```python
from build123d import *

# Parameters (mm, degrees)
SKETCH1_W           = 10
SKETCH1_H           = 10
BOSS_EXTRUDE1_DEPTH = 50
BOSS_EXTRUDE2_START = -45
SKETCH2_R           = 20
BOSS_EXTRUDE2_DEPTH = 2.5
FILLET2_R           = 2
FILLET3_R           = 5
FILLET4_R           = 5


with BuildPart() as part:
    # Sketch1 → Boss-Extrude1 (new, symmetric)
    with BuildSketch(Plane(origin=(0, 0, 0), x_dir=(1, 0, 0), z_dir=(0, 1, 0))):
        Rectangle(SKETCH1_W, SKETCH1_H)
    extrude(amount=BOSS_EXTRUDE1_DEPTH, both=True)

    # Sketch2 → Boss-Extrude2 (add, symmetric)
    with BuildSketch(Plane(origin=(0, 50, 0), x_dir=(1, 0, 0), z_dir=(0, 1, 0)).offset(BOSS_EXTRUDE2_START)):
        with Locations(Location((0, 0, 0), (0, 0, 270))):
            Circle(SKETCH2_R)
    extrude(amount=BOSS_EXTRUDE2_DEPTH, both=True)

    # Fillet2
    fillet2_edges = [part.edges().sort_by_distance(p)[0] for p in [
        (5, -23.75, 5),
        (-5, -23.75, 5),
        (-5, -23.75, -5),
        (5, -23.75, -5),
    ]]
    fillet(fillet2_edges, radius=FILLET2_R)

    # Fillet3
    fillet3_edges = [part.edges().sort_by_distance(p)[0] for p in [
        (-5, 28.75, -5),
        (-5, 28.75, 5),
        (5, 28.75, 5),
        (5, 28.75, -5),
    ]]
    fillet(fillet3_edges, radius=FILLET3_R - 0.0001)  # a hair under: the kernel refuses the full size

    # Fillet4
    fillet4_edges = [part.edges().sort_by_distance(p)[0] for p in [
        (3.535563195, 50, -3.535563195),
        (3.535563195, 50, 3.535563195),
        (-3.535563195, 50, 3.535563195),
        (-3.535563195, 50, -3.535563195),
    ]]
    fillet(fillet4_edges, radius=FILLET4_R - 0.0001)  # a hair under: the kernel refuses the full size


solid = part.part
```
Geometry: final body of the model. Coordinates: model frame, mm. A direction names the side the tool comes from. Round coordinates to 2 decimals unless told otherwise and drop trailing zeros. Write each loop counter-clockwise with the first axis right and the second up, starting at its lowest first coordinate (ties: lowest second). Pieces come first, ordered by that corner, then holes.
Item 1: Section query B-B (x = -16). Return loops of the section in (y, z), plus the area to 3 significant figures.
Item 2: Pin query (flat end, axial travel): P1, Ø1.8, axis at y = -31, z = 0.5, coming from the -X side; P2, Ø6.5, axis at x = -1, y = -13, coming from the -Z side; P3, Ø6.5, axis at y = -19, z = 1, coming from the +X side. Return the tip coordinate at first contact, or that it passes through.
Item 3: Material intervals for L1, parallel to X at y = -8.5, z = -1.5; L2, parallel to Y at x = 12, z = -9, sorted ascending.
Item 4: Set-up query: faces 1 (the face through (-4.43, -24.12, -4.4)), 2 (the face through (-4.43, -23.38, 4.4)), 3 (the face through (0, -23, -5)), 4 (the face through (-5, -23, 0)), 5 (the face through (-4, 26, -3)). Return all of +Z, -Z, +X, -X, +Y, -Y with unobstructed straight access to the full face (end or side cutting, diameter ignored); none if empty.
Item 5: Section query A-A (y = -39). Return loops of the section in (x, z).
Completed:
1. outline: (2.5, -12) - (7.5, -12) - (7.5, 12) - (2.5, 12) - close
1. area: 120 mm2
2. P1: stops at x = -5
2. P2: stops at z = -5
2. P3: stops at x = 5
3. L1: x = -5 to 5
3. L2: y = 2.5 to 7.5
4. face 1: -Z, -X, -Y
4. face 2: +Z, -X, -Y
4. face 3: -Z, +X, -X, -Y
4. face 4: +Z, -Z, -X, -Y
4. face 5: -Z, -X, +Y
5. outline: (-5, -3) arc R2 ccw to (-3, -5) - (3, -5) arc R2 ccw to (5, -3) - (5, 3) arc R2 ccw to (3, 5) - (-3, 5) arc R2 ccw to (-5, 3) - close
